Here's how the part is built. I have some questions about the finished solid (model axes, mm). A direction names the side the tool comes from. Round coordinates to 2 decimals unless told otherwise and drop trailing zeros. Order: outer loops, then holes, each group sorted by start corner. A loop starts at its lowest first (then second) coordinate and runs counter-clockwise, first axis right, second up. Notation, with made-up numbers: (19, 56) - (35, 56) arc R37 ccw to (35, 94) - close; hole circle Ø3 at (45, 24.25). An arc over 180 degrees is marked (long way). Answer as a JSON object with one key per item and string values.
```python
from build123d import *

# Parameters (mm, degrees)
F0_W      = 18.0097855628
F0_H      = 33.7471626699
F1_DEPTH  = 350.012
F2_W      = 17.9832
F2_H      = 279.7042541206
F3_DEPTH  = 33.782
F4_W      = 579.9328
F4_H      = 33.782
F5_DEPTH  = 18.034
F6_W      = 17.9832
F6_H      = 33.782
F7_DEPTH  = 279.908
F8_W      = 580.1614
F8_H      = 33.6901992559
F9_DEPTH  = 18.034
F10_W     = 34.3154
F10_H     = 351.8910109997
F11_DEPTH = 18.034
F12_W     = 33.8344089687
F12_H     = 351.4855802059
F13_DEPTH = 18.034
F14_W     = 34.417
F14_H     = 351.3836
F15_DEPTH = 18.034
F16_W     = 280.7166390121
F16_H     = 34.9791944027
F17_DEPTH = 18.034
F18_W     = 279.0465280414
F18_H     = 34.7275435925
F19_DEPTH = 18.034
F20_W     = 579.12
F20_H     = 34.9791944027
F21_DEPTH = 18.034
F22_W     = 579.882
F22_H     = 34.7275435925
F23_DEPTH = 18.034


with BuildPart() as f1:
    # F0 (on Top) → F1 (new body)
    with BuildSketch(Plane.XY):
        with Locations((-9.0048927814, -16.8735813349)):
            Rectangle(F0_W, F0_H)
    extrude(amount=F1_DEPTH)

    # F2 (on Top) → F3 (join)
    with BuildSketch(Plane.XY):
        with Locations((-26.6942894229, 106.0177180916)):
            Rectangle(F2_W, F2_H)
    extrude(amount=F3_DEPTH)

    # F4 (on face) → F5 (join)
    with BuildSketch(Plane.XZ.offset(33.8344089687)):
        with Locations((254.2805105771, 16.891)):
            Rectangle(F4_W, F4_H)
    extrude(amount=F5_DEPTH)

    # F6 (on face) → F7 (join)
    with BuildSketch(Plane(origin=(0, -33.8344089687, 0), x_dir=(-1, 0, 0), z_dir=(0, 1, 0))):
        with Locations((-535.2553105771, 16.891)):
            Rectangle(F6_W, F6_H)
    extrude(amount=F7_DEPTH)

    # F8 (on face) → F9 (join)
    with BuildSketch(Plane(origin=(0, 245.8698451519, 0), x_dir=(-1, 0, 0), z_dir=(0, 1, 0))):
        with Locations((-254.3948105771, 16.845099628)):
            Rectangle(F8_W, F8_H)
    extrude(amount=F9_DEPTH)

    # F10 (on face) → F11 (join)
    with BuildSketch(Plane.YZ.offset(-17.7026894229)):
        with Locations((228.7121451519, 175.9455054998)):
            Rectangle(F10_W, F10_H)
    extrude(amount=F11_DEPTH)

    # F12 (on face) → F13 (join)
    with BuildSketch(Plane(origin=(526.2637105771, 0, 0), x_dir=(0, -1, 0), z_dir=(-1, 0, 0))):
        with Locations((16.9172044843, 175.742790103)):
            Rectangle(F12_W, F12_H)
    extrude(amount=F13_DEPTH)

    # F14 (on face) → F15 (join)
    with BuildSketch(Plane(origin=(526.2637105771, 0, 0), x_dir=(0, -1, 0), z_dir=(-1, 0, 0))):
        with Locations((-228.2942401447, 175.6918)):
            Rectangle(F14_W, F14_H)
    extrude(amount=F15_DEPTH)

    # F16 (on face) → F17 (join)
    with BuildSketch(Plane(origin=(526.2637105771, 0, 0), x_dir=(0, -1, 0), z_dir=(-1, 0, 0))):
        with Locations((-105.6323889643, 335.1304978132)):
            Rectangle(F16_W, F16_H)
    extrude(amount=-F17_DEPTH)

    # F18 (on face) → F19 (join)
    with BuildSketch(Plane.YZ.offset(-17.7026894229)):
        with Locations((106.0337163508, 334.9141031504)):
            Rectangle(F18_W, F18_H)
    extrude(amount=-F19_DEPTH)

    # F20 (on face) → F21 (join)
    with BuildSketch(Plane(origin=(0, 245.9907084703, 0), x_dir=(-1, 0, 0), z_dir=(0, 1, 0))):
        with Locations((-254.7377105771, 335.1304978132)):
            Rectangle(F20_W, F20_H)
    extrude(amount=F21_DEPTH)

    # F22 (on face) → F23 (join)
    with BuildSketch(Plane.XZ.offset(33.4895476699)):
        with Locations((254.2043105771, 334.9141031504)):
            Rectangle(F22_W, F22_H)
    extrude(amount=F23_DEPTH)


solid = f1.part
```
1. For P1, Ø10, axis at y = 23, z = 15, coming from the +X side; P2, Ø1, axis at y = 216.5, z = 160, coming from the -X side; P3, Ø14.5, axis at x = 516, z = 170, coming from the -Y side, each with a flat end and sliding along its axis, tell me the tip position at first contact or that it passes through.
Responses:
{"P1": "x = 544.25", "P2": "x = -17.7", "P3": "y = -33.83"}
2. Imagine slicing it at C-C (x = 361). List the corners of the cut face in (y, z) for me.
Responses:
{"outline": "(-51.87, 0) - (-33.83, 0) - (-33.83, 33.78) - (-51.87, 33.78) - close; (-51.52, 317.55) - (-33.49, 317.55) - (-33.49, 352.28) - (-51.52, 352.28) - close; (245.87, 0) - (263.9, 0) - (263.9, 33.69) - (245.87, 33.69) - close; (245.99, 317.64) - (264.02, 317.64) - (264.02, 352.62) - (245.99, 352.62) - close"}
3. Imagine slicing it at A-A (y = -11). List the corners of the cut face in (x, z) for me.
Responses:
{"outline": "(-35.74, 317.55) - (-18.01, 317.55) - (-18.01, 33.78) - (-35.69, 33.78) - (-35.69, 0) - (0, 0) - (0, 350.01) - (-17.7, 350.01) - (-17.7, 352.28) - (-35.74, 352.28) - close; (508.23, 0) - (544.25, 0) - (544.25, 33.78) - (526.26, 33.78) - (526.26, 317.64) - (544.3, 317.64) - (544.3, 352.62) - (526.26, 352.62) - (526.26, 351.49) - (508.23, 351.49) - close"}
4. Imagine slicing it at B-B (z = 306.5). List the corners of the cut face in (x, y) for me.
Responses:
{"outline": "(-18.01, -33.75) - (0, -33.75) - (0, 0) - (-18.01, 0) - close; (-17.7, 211.55) - (0.33, 211.55) - (0.33, 245.87) - (-17.7, 245.87) - close; (508.23, -33.83) - (526.26, -33.83) - (526.26, 0) - (508.23, 0) - close; (508.23, 211.09) - (526.26, 211.09) - (526.26, 245.5) - (508.23, 245.5) - close"}
5. If I drill on L1, parallel to Y at x = 511, z = 336.5; L2, parallel to X at y = 222, z = 245.5; L3, parallel to X at y = 3, z = 335, over which ranges is the centre line in solid material (lowest first)? Write a range as [from, to].
Responses:
{"L1": "[-51.52, 0], [211.09, 245.5], [245.99, 264.02]", "L2": "[-17.7, 0.33], [508.23, 526.26]", "L3": "[-35.74, -17.7], [526.26, 544.3]"}
6. For faces 5 (the face through (-17.703, 104, 17)), 6 (the face through (517, 229, 351.384)), which set-ups out of +Z, -Z, +X, -X, +Y, -Y let a thin tool reach every point of the face, with its end or its side?
Responses:
{"face 5": "+Z, -Z", "face 6": "+Z"}
7. Thinking about a two-plate mould opening in Y: for faces 1 (the face through (517, 0, 173)), 2 (the face through (526.264, 229, 178)), 3 (the face through (-17.703, 104, 335)), 4 (the face through (250, -51.524, 335)), which applies, pulls with the +Y half, pulls with the -Y half, needs draft (parallel to the pull), parting line crosses it, or undercut?
Responses:
{"face 1": "undercut", "face 2": "needs draft", "face 3": "undercut", "face 4": "pulls with the -Y half"}
